The listing builds one solid part. Answer for the finished solid, in the listing's coordinates (mm). Give positions to 0.01 mm unless a question says otherwise; leave off trailing zeros. Write each loop counter-clockwise with the first axis right and the second up, starting at its lowest first coordinate (ties: lowest second). Pieces come first, ordered by that corner, then holes. Notation, with made-up numbers: (-36, 12.5) - (-9, 12.5) arc R6 ccw to (-9, 22.5) - close; hole circle Ø10 at (-31, 65.25). An arc over 180 degrees is marked (long way). Use a Markdown table: item, result. Add a question column.
from build123d import *

# Parameters (mm, degrees)
F0_W     = 12
F0_H     = 30
F1_DEPTH = 8
F2_R     = 4
F3_DEPTH = 8.001
F5_D     = 2.5


with BuildPart() as f1:
    # F0 (on Top) → F1 (new body)
    with BuildSketch(Plane.XY):
        Rectangle(F0_W, F0_H)
    extrude(amount=F1_DEPTH)

    # F2 (on Top) → F3 (cut, through all)
    with BuildSketch(Plane.XY):
        Circle(F2_R)
    extrude(amount=F3_DEPTH, mode=Mode.SUBTRACT)

    # F5 (through all)
    with Locations(Plane(origin=(0, 0, 0), x_dir=(1, 0, 0), z_dir=(0, 0, -1))):
        with Locations((0, -9), (0, 9)):
            Hole(F5_D / 2)


solid = f1.part
1. For a pull along Y with two mould halves and no side action, classify faces 1 (the cylindrical face through (-0.867, -3.905, 3.944)), 2 (the flat face through (0, -15, 4)), 3 (the flat face through (-3, 4, 0)) as released by +Y, released by -Y, zero draft, split by the parting line, or undercut.
2. The part is cut by section A-A (x = 0). Give the vertices of the cut face in (y, z).
3. The part is cut by section D-D (x = -2.5). Give the vertices of the cut face in (y, z), and give its area (3 significant figures).
4. Consider L1, parallel to Y at x = 0, z = 2; L2, parallel to X at y = 9, z = 4.25; L3, parallel to Y at x = 1, z = 1. Determine where each line is inside the solid, lowest interval first. Write a range as [from, to].
5. The part is cut by section B-B (y = 9). Give the vertices of the cut face in (x, z), and give its area (3 significant figures).
6. The part is cut by section C-C (z = 1.75). Give the vertices of the cut face in (x, y), and give its area (3 significant figures).
Check values:
| question | item | result |
|---|---|---|
| 1 | face 1 | undercut |
| 1 | face 2 | released by -Y |
| 1 | face 3 | zero draft |
| 2 | outline | (-15, 0) - (-10.25, 0) - (-10.25, 8) - (-15, 8) - close; (-7.75, 0) - (-4, 0) - (-4, 8) - (-7.75, 8) - close; (4, 0) - (7.75, 0) - (7.75, 8) - (4, 8) - close; (10.25, 0) - (15, 0) - (15, 8) - (10.25, 8) - close |
| 3 | outline | (-15, 0) - (-3.12, 0) - (-3.12, 8) - (-15, 8) - close; (3.12, 0) - (15, 0) - (15, 8) - (3.12, 8) - close |
| 3 | area | 190 mm2 |
| 4 | L1 | y = [-15, -10.25], [-7.75, -4], [4, 7.75], [10.25, 15] |
| 4 | L2 | x = [-6, -1.25], [1.25, 6] |
| 4 | L3 | y = [-15, -9.75], [-8.25, -3.87], [3.87, 8.25], [9.75, 15] |
| 5 | outline | (-6, 0) - (-1.25, 0) - (-1.25, 8) - (-6, 8) - close; (1.25, 0) - (6, 0) - (6, 8) - (1.25, 8) - close |
| 5 | area | 76.0 mm2 |
| 6 | outline | (-6, -15) - (6, -15) - (6, 15) - (-6, 15) - close; hole circle Ø8 at (0, 0); hole circle Ø2.5 at (0, -9); hole circle Ø2.5 at (0, 9) |
| 6 | area | 300 mm2 |
